CAD build for the part. Positions are in the model's coordinates, mm. A direction names the side the tool comes from. Round coordinates to 2 decimals unless told otherwise and drop trailing zeros. Order: outer loops, then holes, each group sorted by start corner. A loop starts at its lowest first (then second) coordinate and runs counter-clockwise, first axis right, second up. Notation, with made-up numbers: (89, 42) - (122, 42) arc R25 cw to (122, 80) - close; hole circle Ø4 at (21, -21.5). An arc over 180 degrees is marked (long way). Write item = value, one per line.
from build123d import *

# Parameters (mm, degrees)
F1_DEPTH = 8
F2_R     = 1.5
F3_DEPTH = 8.001
F4_R     = 28.523991
F5_R     = 5


with BuildPart() as f1:
    # F0 (on Top) → F1 (new body)
    with BuildSketch(Plane.XY):
        with BuildLine():
            ThreePointArc((-53.434796, -180.246283), (-157.807923, -102.179545), (-186.330352, 25))
            Line((-186.330352, 25), (-208.506595, 25))
            ThreePointArc((-208.506595, 25), (0, -210), (208.506595, 25))
            Line((208.506595, 25), (186.330352, 25))
            ThreePointArc((186.330352, 25), (157.807923, -102.179545), (53.434796, -180.246283))
            Line((53.434796, -180.246283), (25, -168))
            Line((25, -168), (0, -168))
            Line((0, -168), (-25, -168))
            Line((-25, -168), (-53.434796, -180.246283))
        make_face()
    extrude(amount=F1_DEPTH)

    # F2 (on face) → F3 (cut, through all)
    with BuildSketch(Plane.XY.offset(8)):
        with Locations((-61.492936, -189.111742)):
            Circle(F2_R)
        with Locations((-116.970716, -160.851562)):
            Circle(F2_R)
        with Locations((-161.000343, -116.830956)):
            Circle(F2_R)
        with Locations((-189.271892, -61.35897)):
            Circle(F2_R)
        with Locations((-199.017947, 0.134414)):
            Circle(F2_R)
        with Locations((61.495827, -189.09914)):
            Circle(F2_R)
        with Locations((116.967814, -160.827591)):
            Circle(F2_R)
        with Locations((160.988419, -116.797963)):
            Circle(F2_R)
        with Locations((189.248599, -61.320184)):
            Circle(F2_R)
        with Locations((198.982051, 0.175196)):
            Circle(F2_R)
        with Locations((-21, -175.002152)):
            Circle(F2_R)
        with Locations((-40.990327, -194.449982)):
            Circle(F2_R)
        with Locations((-10.202835, -198.738276)):
            Circle(F2_R)
        with Locations((21, -174.997848)):
            Circle(F2_R)
        with Locations((10.2077, -198.736184)):
            Circle(F2_R)
        with Locations((40.994312, -194.441581)):
            Circle(F2_R)
    extrude(amount=-F3_DEPTH, mode=Mode.SUBTRACT)

    # F4
    f4_edges = [f1.edges().sort_by_distance(p)[0] for p in [
        (25, -168, 4),
        (-25, -168, 4),
    ]]
    fillet(f4_edges, radius=F4_R)

    # F5
    f5_edges = [f1.edges().sort_by_distance(p)[0] for p in [
        (53.434796, -180.246283, 4),
        (-53.434796, -180.246283, 4),
    ]]
    fillet(f5_edges, radius=F5_R)


solid = f1.part
(1) Band-saw the part on B-B on x = 0. List the corners of the cut face in (y, z).
Solved:
outline = (-210, 0) - (-168, 0) - (-168, 8) - (-210, 8) - close
(2) Band-saw the part on A-A on z = 3. Count the separate pieces of the cut face and the enclosed holes in it, plus the area to 3 significant figures.
Solved:
separate_pieces = 1
enclosed_holes = 16
area = 16,300 mm²
(3) Tool access for faces 1 (the cylindrical face through (-157.3, -102.96, 3.94)), 2 (the flat face through (-197, 25, 4)), 3 (the cylindrical face through (-24.958, -168.604, 4.056)): list every direction of +Z, -Z, +X, -X, +Y, -Y with a clear straight run to the whole face (end or side of a thin tool).
Solved:
face_1 = +Z, -Z
face_2 = +Z, -Z, +X, -X, +Y
face_3 = +Z, -Z, +Y
(4) Pull direction X, two halves, no side cores. Call faces 4 (the flat face through (0, -168, 4)), 5 (the cylindrical face through (-4.97, -209.94, 3.94)), 6 (the flat face through (-1, -170, 0)): released by +X, released by -X, zero draft, split by the parting line, or undercut.
Solved:
face_4 = undercut
face_5 = split by the parting line
face_6 = zero draft
(5) Probe line 1 along X through (y, z) = (-190, 5.75); line 2 along X through (y, z) = (-137, 7); line 3 along X through (y, z) = (-1, 7.25). List the from-to ranges inside material, lowest first.
Solved:
line_1 = -89.44 to -62.7, -60.28 to 60.3, 62.7 to 89.44
line_2 = -159.16 to -128.74, 128.74 to 159.16
line_3 = -210 to -200, -198.04 to -188, 188 to 198.05, 199.91 to 210
(6) Band-saw the part on C-C on x = 77.5. List the corners of the cut face in (y, z).
Solved:
outline = (-195.18, 0) - (-171.28, 0) - (-171.28, 8) - (-195.18, 8) - close
(7) Drop flat-ended pins along their axis: pin 1 (2.5 mm diameter, centred on x = -40.99, y = -194.45, fed in from -Z); pin 2 (2 mm diameter, centred on x = -121.5, z = 4.5, fed in from +Y); pin 3 (4 mm diameter, centred on x = -78.5, z = 6.5, fed in from -Y); pin 4 (1 mm diameter, centred on y = -113, z = 3.5, fed in from -X). Give the stop position or say it passes through.
Solved:
pin_1 = through
pin_2 = -142.61
pin_3 = -195.57
pin_4 = -177.32
